For this review, take the finished solid that the model builds, in its own axes (mm). A direction names the side the tool comes from. Give positions to 0.01 mm unless a question says otherwise; leave off trailing zeros. Write each loop counter-clockwise with the first axis right and the second up, starting at its lowest first coordinate (ties: lowest second). Pieces come first, ordered by that corner, then holes. Notation, with made-up numbers: M 88.25,68.5 L 112.25,68.5 A21 ccw 112.25,92.5 Z; hole C -4.5,88 d8. An arc over 180 degrees is marked long. Write item = value, one per line.
```python
from build123d import *

# Parameters (mm, degrees)
F0_W                  = 34.2
F0_H                  = 34.2
F0_W_2                = 28.2
F0_H_2                = 28.2
F1_DEPTH              = 3
F2_DEPTH              = 31.2
F3_W                  = 34.2
F3_H                  = 34.2
F3_W_2                = 28.2
F3_H_2                = 28.2
F4_DEPTH              = 31.2
F5_W                  = 34.2
F5_H                  = 34.2
F5_W_2                = 28.2
F5_H_2                = 28.2
F6_DEPTH              = 31.2
F7_D                  = 3.3
F7_DEPTH              = 13.5
F7_CSINK_D            = 6.72
F7_CSINK_ANGLE        = 90
F7_TIP                = 0.9914200214
F7_ON_F3_D            = 3.3
F7_ON_F3_DEPTH        = 13.5
F7_ON_F3_CSINK_D      = 6.72
F7_ON_F3_CSINK_ANGLE  = 90
F7_ON_F3_TIP          = 0.9914200214
F10_D                 = 3.3
F10_DEPTH             = 13.5
F10_CSINK_D           = 6.72
F10_CSINK_ANGLE       = 90
F10_TIP               = 0.9914200214
F10_ON_F8_D           = 3.3
F10_ON_F8_DEPTH       = 13.5
F10_ON_F8_CSINK_D     = 6.72
F10_ON_F8_CSINK_ANGLE = 90
F10_ON_F8_TIP         = 0.9914200214
F12_DEPTH             = 34.2
F13_R                 = 5
F14_R                 = 1.49999
F15_D                 = 5.5


# Not quite as in the source:
# - a fillet or chamfer is up to 0.001 mm smaller than in the source, because OpenCascade refuses the exact size


with BuildPart() as f1:
    # F0 (on Top) → F1 (new body)
    with BuildSketch(Plane.XY):
        with Locations((-14.1, 14.1)):
            Rectangle(F0_W, F0_H)
        with Locations((-14.1, 14.1)):
            Rectangle(F0_W_2, F0_H_2, mode=Mode.SUBTRACT)
        with Locations((-14.1, 14.1)):
            Rectangle(F0_W_2, F0_H_2)
    extrude(amount=-F1_DEPTH)

    # F0 (on Top) → F2 (join)
    with BuildSketch(Plane.XY):
        with Locations((-14.1, 14.1)):
            Rectangle(F0_W, F0_H)
        with Locations((-14.1, 14.1)):
            Rectangle(F0_W_2, F0_H_2, mode=Mode.SUBTRACT)
    extrude(amount=F2_DEPTH)

    # F3 (on face) → F4 (join)
    with BuildSketch(Plane.XZ.offset(3)):
        with Locations((-14.1, 14.1)):
            Rectangle(F3_W, F3_H)
        with Locations((-14.1, 14.1)):
            Rectangle(F3_W_2, F3_H_2, mode=Mode.SUBTRACT)
    extrude(amount=F4_DEPTH)

    # F5 (on face) → F6 (join)
    with BuildSketch(Plane.YZ.offset(3)):
        with Locations((14.1, 14.1)):
            Rectangle(F5_W, F5_H)
        with Locations((14.1, 14.1)):
            Rectangle(F5_W_2, F5_H_2, mode=Mode.SUBTRACT)
    extrude(amount=F6_DEPTH)

    # F7
    with Locations(Plane.YZ.offset(3)):
        with Locations((14.1, 14.1)):
            CounterSinkHole(F7_D / 2, F7_CSINK_D / 2, depth=F7_DEPTH, counter_sink_angle=F7_CSINK_ANGLE)
            with Locations((0, 0, -(F7_DEPTH + F7_TIP / 2))):  # 118° drill point
                Cone(0, F7_D / 2, F7_TIP, mode=Mode.SUBTRACT)

    # F7 on F3
    with Locations(Plane.XZ.offset(3)):
        with Locations((-14.1, 14.1)):
            CounterSinkHole(F7_ON_F3_D / 2, F7_ON_F3_CSINK_D / 2, depth=F7_ON_F3_DEPTH, counter_sink_angle=F7_ON_F3_CSINK_ANGLE)
            with Locations((0, 0, -(F7_ON_F3_DEPTH + F7_ON_F3_TIP / 2))):  # 118° drill point
                Cone(0, F7_ON_F3_D / 2, F7_ON_F3_TIP, mode=Mode.SUBTRACT)

    # F10
    with Locations(Plane.XZ.offset(3)):
        with Locations((17.85, 14.1)):
            CounterSinkHole(F10_D / 2, F10_CSINK_D / 2, depth=F10_DEPTH, counter_sink_angle=F10_CSINK_ANGLE)
            with Locations((0, 0, -(F10_DEPTH + F10_TIP / 2))):  # 118° drill point
                Cone(0, F10_D / 2, F10_TIP, mode=Mode.SUBTRACT)

    # F10 on F8
    with Locations(Plane.YZ.offset(3)):
        with Locations((-17.85, 14.1)):
            CounterSinkHole(F10_ON_F8_D / 2, F10_ON_F8_CSINK_D / 2, depth=F10_ON_F8_DEPTH, counter_sink_angle=F10_ON_F8_CSINK_ANGLE)
            with Locations((0, 0, -(F10_ON_F8_DEPTH + F10_ON_F8_TIP / 2))):  # 118° drill point
                Cone(0, F10_ON_F8_D / 2, F10_ON_F8_TIP, mode=Mode.SUBTRACT)

    # F11 (on face) → F12 (join, through all)
    with BuildSketch(Plane.XY.offset(31.2)):
        with BuildLine():
            Line((-31.2, 0), (-35.2, 0))
            ThreePointArc((-35.2, 0), (-39.2, -4), (-35.2, -8))
            Line((-35.2, -8), (-31.2, -8))
            Line((-31.2, -8), (-31.2, 0))
        make_face()
    extrude(amount=-F12_DEPTH)

    # F13
    f13_edges = [f1.edges().sort_by_distance(p)[0] for p in [
        (-31.2, 0, 14.1),
        (-31.2, -8, 14.1),
    ]]
    fillet(f13_edges, radius=F13_R)

    # F14 (radius 1.5 in the source; OpenCascade refuses exactly that, so slightly less here)
    f14_edges = [f1.edges().sort_by_distance(p)[0] for p in [
        (-32.47322, -9.610939, -3),
        (-32.47322, -9.610939, 31.2),
        (1.5, 31.2, -3),
        (34.2, 31.2, 14.1),
        (1.5, 31.2, 31.2),
        (-31.2, 31.2, 14.1),
        (-31.2, -34.2, 14.1),
        (-14.1, -34.2, -3),
        (3, -34.2, 14.1),
        (-14.1, -34.2, 31.2),
        (-14.1, -34.2, 28.2),
        (0, -34.2, 14.1),
        (-14.1, -34.2, 0),
        (-28.2, -34.2, 14.1),
        (3, -18.6, -3),
        (3, -3, 14.1),
        (18.6, -3, -3),
        (3, -18.6, 31.2),
        (18.6, -3, 31.2),
        (34.2, -3, 14.1),
        (34.2, 14.1, -3),
        (34.2, 28.2, 14.1),
        (34.2, 14.1, 28.2),
        (34.2, 14.1, 31.2),
        (34.2, 14.1, 0),
        (34.2, 0, 14.1),
        (-14.1, 0, 31.2),
        (-28.2, 14.1, 31.2),
        (-14.1, 28.2, 31.2),
        (0, 0, 15.6),
        (-31.2, 18.072136, 31.2),
        (-31.2, 18.072136, -3),
        (-31.2, -23.572136, 31.2),
        (-39.2, -4, 31.2),
        (-32.47322, 1.610939, 31.2),
        (0, 14.1, 31.2),
        (-32.47322, 1.610939, -3),
        (-39.2, -4, -3),
        (-31.2, -23.572136, -3),
    ]]
    fillet(f14_edges, radius=F14_R)

    # F15 (through all)
    with Locations(Plane.XY.offset(31.2)):
        with Locations((-35.2, -4)):
            Hole(F15_D / 2)


solid = f1.part
```
1. We need section C-C, the plane x = 8.5. Write out the cut boundary in (y, z).
Responses:
outline = M -3,-1.5 A1.5 ccw -1.5,-3 L 29.7,-3 A1.5 ccw 31.2,-1.5 L 31.2,29.7 A1.5 ccw 29.7,31.2 L -1.5,31.2 A1.5 ccw -3,29.7 Z; hole M 0,0 L 28.2,0 L 28.2,28.2 L 0,28.2 Z
2. We need section D-D, the plane y = -17.85. Write out the cut boundary in (x, z).
Responses:
outline = M -31.2,-1.5 A1.5 ccw -29.7,-3 L 1.5,-3 A1.5 ccw 3,-1.5 L 3,10.74 L 1.29,12.45 L 0,12.45 L 0,0 L -28.2,0 L -28.2,28.2 L 0,28.2 L 0,15.75 L 1.29,15.75 L 3,17.46 L 3,29.7 A1.5 ccw 1.5,31.2 L -29.7,31.2 A1.5 ccw -31.2,29.7 Z
3. The part is to be moulded in two halves that separate along Y. For faces 1 (the face through (0.64, -16.54, 13.1)), 2 (the face through (-1, -2, 31.2)), 3 (the face through (18, 14, 0)), 4 (the face through (-17, -3, 17)), say which applies: +Y half, -Y half, draft (parallel to the pull), parting line (faces both ways), or undercut.
Responses:
face_1 = undercut
face_2 = draft
face_3 = undercut
face_4 = -Y half
4. Insertion check: P1, Ø6, axis at x = -25.5, z = 19, coming from the -Y side; P2, Ø14, axis at x = -15.5, z = 13, coming from the -Y side; P3, Ø14, axis at y = -20.5, z = 12.5, coming from the -X side; P4, Ø3.5, axis at x = -35.2, y = -4, coming from the +Z side. Each pin has a flat end and moves straight along its axis. Give the tip position at first contact, or say it passes through.
Responses:
P1 = -33.6
P2 = -3
P3 = -31.2
P4 = through
5. Machinability: for faces 5 (the face through (18, 14, 28.2)), 6 (the face through (-31.2, -23, 14)), 7 (the face through (22, -3, 14)), 8 (the face through (-31.2, 17, 14)), 9 (the face through (0, 12, 15)), which of the approach directions +Z, -Z, +X, -X, +Y, -Y give a long, thin tool a straight path to every point of the face, cutting with its end or side? Answer none if there is none.
Responses:
face_5 = +X
face_6 = +Z, -Z, -X, -Y
face_7 = +Z, -Z, +X, -Y
face_8 = +Z, -Z, -X, +Y
face_9 = +Z
6. For line 1 along X through (y, z) = (-14.5, 10); line 2 along Y through (x, z) = (-11, 19.5), list the stretches that pass through material, from the lowest coordinate up. Write a range as from..to.
Responses:
line_1 = -31.2..-28.2, 0..3
line_2 = -3..0, 28.2..31.2
